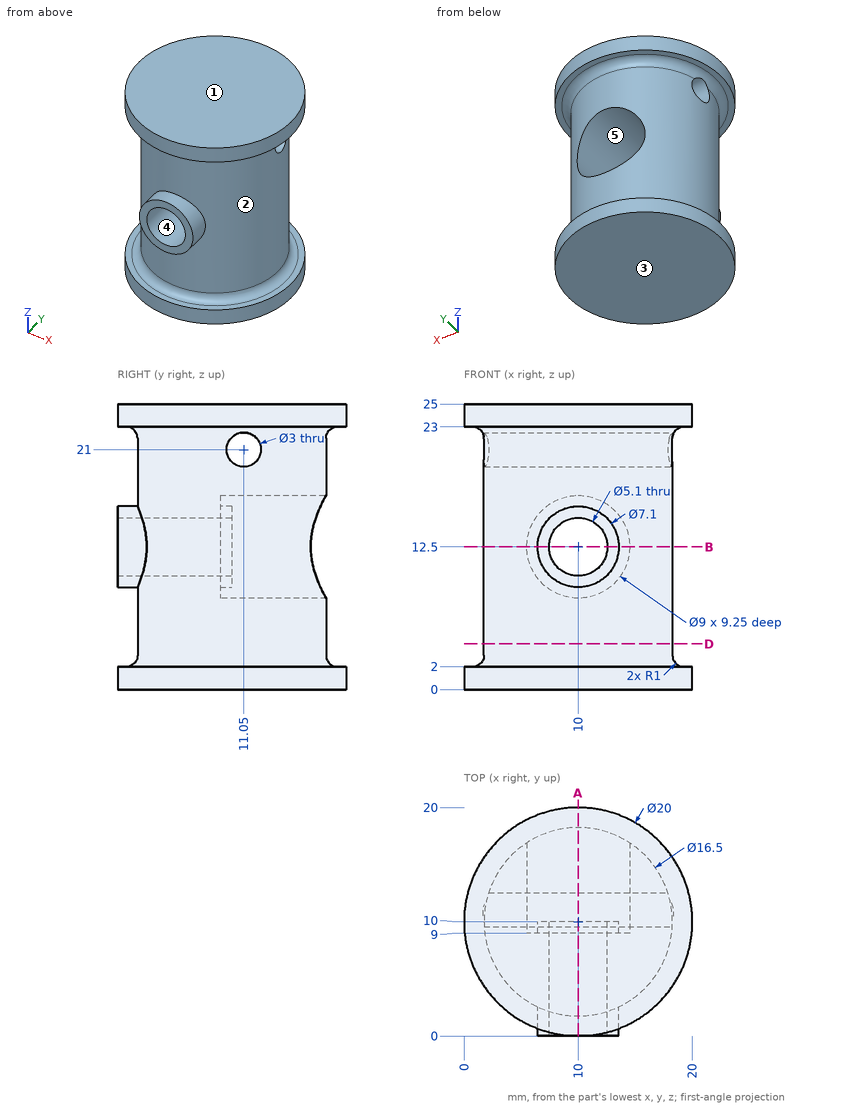
Drawing for the job (mm, zero at the part's lowest x, y, z). A direction names the side the tool comes from. Round coordinates to 2 decimals unless told otherwise and drop trailing zeros. Write each loop counter-clockwise with the first axis right and the second up, starting at its lowest first coordinate (ties: lowest second). Pieces come first, ordered by that corner, then holes. Notation, with made-up numbers: (54.5, 89.5) - (66.5, 89.5) arc R12 ccw to (66.5, 108.5) - close; hole circle Ø7 at (69.5, 61.5). An arc over 180 degrees is marked (long way). Write item = value, one per line. Start each with the question number.
Q1. Band-saw the part on A-A (x = 10). Count the separate pieces of the cut face and the enclosed holes in it, then the cut area to 3 significant figures.
Q2. Drop flat-ended pins along their axis: pin 1 (1 mm diameter, centred on x = 16.5, z = 9, fed in from -Y); pin 2 (4 mm diameter, centred on x = 16, z = 21.5, fed in from +Y); pin 3 (4.5 mm diameter, centred on x = 11.5, z = 14, fed in from +Y); pin 4 (4 mm diameter, centred on x = 10, z = 12.5, fed in from +Y). Give the stop position or say it passes through.
Q3. Which spindle directions (+Z, -Z, +X, -X, +Y, -Y) get a long thin tool onto all of the face, cutting with end or side? Do the marked faces 4 and 5. Say none if no direction does.
Q4. Band-saw the part on B-B (z = 12.5). Give the cut face in (x, y).
Q5. Probe L1, parallel to Z at x = 11.75, y = 11.05; L2, parallel to Z at x = 1.25, y = 13.5; L3, parallel to Z at x = 12, y = 9.75. List the from-to ranges inside material, lowest first. Write a range as from..to.
Q6. Mould opens along Z. For the marked faces 1, 2 and 3 say: pulls with the +Z half, pulls with the -Z half, needs draft (parallel to the pull), parting line crosses it, or undercut.
Q7. Band-saw the part on D-D (z = 4). Give the cut face in (x, y).
Answers below:
q1.separate_pieces = 2
q1.enclosed_holes = 1
q1.area = 306 mm2
q2.pin_1 = 4.34
q2.pin_2 = 18.84
q2.pin_3 = 10
q2.pin_4 = through
q3.face_4 = +Y, -Y
q3.face_5 = +Y
q4.outline = (5.5, 9) - (5.5, 16.91) arc R8.25 ccw to (6.45, 2.55) - (6.45, 0) - (7.45, 0) - (7.45, 10) - (6.45, 10) - (6.45, 9) - close; (12.55, 0) - (13.55, 0) - (13.55, 2.55) arc R8.25 ccw to (14.5, 16.91) - (14.5, 9) - (13.55, 9) - (13.55, 10) - (12.55, 10) - close
q5.L1 = 0..8.35, 16.65..19.5, 22.5..25
q5.L2 = 0..2, 23..25
q5.L3 = 0..8.47, 9.57..10.92, 14.08..15.43, 16.53..20.25, 21.75..25
q6.face_1 = pulls with the +Z half
q6.face_2 = undercut
q6.face_3 = pulls with the -Z half
q7.outline = circle Ø16.5 at (10, 10)
